Model file for the job. Use its own axes, mm. A direction names the side the tool comes from. Round coordinates to 2 decimals unless told otherwise and drop trailing zeros. Loops run counter-clockwise (first coordinate to the right, second up) from the corner with the lowest first, then second, coordinate; pieces in that order, holes last. Notation, with made-up numbers: M 76,25 L 134,25 A28 cw 134,47 Z; hole C -11.75,-15 d9. An arc over 180 degrees is marked long. Use a Markdown table: item, result. Add a question column.
Item 1: Tool access for faces 4 (the flat face through (-4, -17, 12.065)), 5 (the flat face through (-1, -16, 15.875)): list every direction of +Z, -Z, +X, -X, +Y, -Y with a clear straight run to the whole face (end or side of a thin tool).
Item 2: Wall check: L1, parallel to Y at x = 39.5, z = 6 (3 decimals); L2, parallel to Z at x = -63.5, y = -31.55 (3 decimals); L3, parallel to Z at x = 8, y = -27 (3 decimals). Give the ranges that are in metal, low to high. Write a range as from..to.
Item 3: Pin check, flat tip, straight feed: P1, Ø1.5, axis at x = 1, y = -8, coming from the -Z side (3 decimals). Stop position of the tip, or through.
Item 4: Saw through at D-D on z = -12. Write the cut outline in (x, y) (3 decimals), then the cut area to 3 significant figures.
Item 5: Saw through at A-A on x = -63.5. Write the cut outline in (y, z) (3 decimals).
Item 6: Saw through at B-B on z = 1.5. Write the cut outline in (x, y) (3 decimals), then the cut area to 3 significant figures.
Item 7: Saw through at C-C on y = -10. Write the cut outline in (x, z) (3 decimals), then the cut area to 3 significant figures.
Item 8: Two-plate mould, pull along Z, no slides. Class faces 1 (the flat face through (11, -30, -15.875)), 2 (the cylindrical face through (-69.844, -31.41, -2.896)), 3 (the flat face through (-1, 0, 0)): +Z half, -Z half, draft (parallel to the pull), parting line (faces both ways), or undercut.
```python
from build123d import *

# Parameters (mm, degrees)
F0_W     = 152.4
F0_H     = 31.75
F0_R     = 6.35
F1_DEPTH = 33.02
F2_W     = 146.05
F2_H     = 26.67
F3_DEPTH = 27.94


with BuildPart() as f1:
    # F0 (on Front) → F1 (new body)
    with BuildSketch(Plane.XZ):
        Rectangle(F0_W, F0_H)
        with Locations((-63.5, -3.175)):
            Circle(F0_R, mode=Mode.SUBTRACT)
    extrude(amount=F1_DEPTH)

    # F2 (on face) → F3 (cut)
    with BuildSketch(Plane(origin=(0, 0, -15.875), x_dir=(1, 0, 0), z_dir=(0, 0, -1))):
        with Locations((-3.175, 16.51)):
            Rectangle(F2_W, F2_H)
    extrude(amount=-F3_DEPTH, mode=Mode.SUBTRACT)


solid = f1.part
```
Entries:
| question | item | result |
|---|---|---|
| 1 | face 4 | -Z, -X |
| 1 | face 5 | +Z, +X, -X, +Y, -Y |
| 2 | L1 | -33.02..-29.845, -3.175..0 |
| 2 | L2 | -15.875..-9.525, 3.175..15.875 |
| 2 | L3 | 12.065..15.875 |
| 3 | P1 | z = 12.065 |
| 4 | outline | M -76.2,-33.02 L 76.2,-33.02 L 76.2,0 L -76.2,0 L -76.2,-3.175 L 69.85,-3.175 L 69.85,-29.845 L -76.2,-29.845 Z |
| 4 | area | 1,140 mm2 |
| 5 | outline | M -33.02,-15.875 L -29.845,-15.875 L -29.845,-9.525 L -33.02,-9.525 Z; M -33.02,3.175 L -29.845,3.175 L -29.845,12.065 L -3.175,12.065 L -3.175,3.175 L 0,3.175 L 0,15.875 L -33.02,15.875 Z; M -3.175,-15.875 L 0,-15.875 L 0,-9.525 L -3.175,-9.525 Z |
| 6 | outline | M -76.2,-33.02 L -67.797,-33.02 L -67.797,-29.845 L -76.2,-29.845 Z; M -76.2,-3.175 L -67.797,-3.175 L -67.797,0 L -76.2,0 Z; M -59.203,-33.02 L 76.2,-33.02 L 76.2,0 L -59.203,0 L -59.203,-3.175 L 69.85,-3.175 L 69.85,-29.845 L -59.203,-29.845 Z |
| 6 | area | 1,080 mm2 |
| 7 | outline | M -76.2,12.065 L 69.85,12.065 L 69.85,-15.875 L 76.2,-15.875 L 76.2,15.875 L -76.2,15.875 Z |
| 7 | area | 758 mm2 |
| 8 | face 1 | -Z half |
| 8 | face 2 | undercut |
| 8 | face 3 | draft |
